Geometry: final body of the model. Coordinates: model frame, mm. Round coordinates to 2 decimals unless told otherwise and drop trailing zeros. Order: outer loops, then holes, each group sorted by start corner. A loop starts at its lowest first (then second) coordinate and runs counter-clockwise, first axis right, second up. Notation, with made-up numbers: (89, 1.25) - (143, 1.25) arc R23 ccw to (143, 32.25) - close; hole circle Ø9 at (-20.75, 11). An arc over 180 degrees is marked (long way). Put each result on its own line as item: value. Start each with the question number.
(1) Pin query (flat end, axial travel): P1, Ø12, axis at y = 0, z = 9, coming from the -X side; P2, Ø10, axis at y = 8.5, z = 65.5, coming from the -X side. Return the tip coordinate at first contact, or that it passes through.
(2) Section C-C (z = 9). Output: boundary loops of the cut face in (x, y).
(3) Material intervals for L1, parallel to Y at x = 3.5, z = -61; L2, parallel to Z at x = 5.5, y = -32.5; L3, parallel to Y at x = 6.5, z = 9, sorted ascending. Write a range as [from, to].
(4) Pull-direction query (Y, two-part tool) for faces 1 (the face through (4.93, -38.58, -53.06)), 2 (the face through (5, 0, 19)), 3 (the face through (0, 14, 1)), 4 (the face through (5, 60, 1)); classes: released by +Y, released by -Y, zero draft, split by the parting line, or undercut.
(5) Section D-D (x = 5.5). Output: boundary loops of the cut face in (y, z), and give its area (3 significant figures).
(6) Section A-A (z = -61). Output: boundary loops of the cut face in (x, y).
(7) Section B-B (y = 32.5). Output: boundary loops of the cut face in (x, z), and give its area (3 significant figures).
from build123d import *

# Parameters (mm, degrees)
SKETCH1_W               = 172
SKETCH1_H               = 120
BOSS_EXTRUDE1_DEPTH     = 10
CUT_EXTRUDE1_DEPTH      = 106.337552658
CUT_EXTRUDE1_DEPTH_BACK = 106.337552658
SKETCH2_R               = 10


with BuildPart() as part:
    # Sketch1 → Boss-Extrude1 (new body)
    with BuildSketch(Plane(origin=(0, 0, 0), x_dir=(0, 0, -1), z_dir=(1, 0, 0))):
        Rectangle(SKETCH1_W, SKETCH1_H)
    extrude(amount=BOSS_EXTRUDE1_DEPTH)

    # Sketch2 → Cut-Extrude1 (cut, two sides: drawn at the far end of the back side and taken through both)
    with BuildSketch(Plane(origin=(10, 0, 0), x_dir=(0, 0, -1), z_dir=(1, 0, 0)).offset(-CUT_EXTRUDE1_DEPTH_BACK)):
        with Locations((-9, 0)):
            Circle(SKETCH2_R)
        with Locations((61, 32.5)):
            Circle(SKETCH2_R)
        with Locations((61, -32.5)):
            Circle(SKETCH2_R)
    extrude(amount=CUT_EXTRUDE1_DEPTH + CUT_EXTRUDE1_DEPTH_BACK, mode=Mode.SUBTRACT)


solid = part.part
Checks:
1. P1: passes through
1. P2: stops at x = 0
2. outline: (0, -60) - (10, -60) - (10, -10) - (0, -10) - close; (0, 10) - (10, 10) - (10, 60) - (0, 60) - close
3. L1: y = [-60, -42.5], [-22.5, 22.5], [42.5, 60]
3. L2: z = [-86, -71], [-51, 86]
3. L3: y = [-60, -10], [10, 60]
4. face 1: undercut
4. face 2: undercut
4. face 3: zero draft
4. face 4: released by +Y
5. outline: (-60, -86) - (60, -86) - (60, 86) - (-60, 86) - close; hole circle Ø20 at (-32.5, -61); hole circle Ø20 at (0, 9); hole circle Ø20 at (32.5, -61)
5. area: 19,700 mm²
6. outline: (0, -60) - (10, -60) - (10, -42.5) - (0, -42.5) - close; (0, -22.5) - (10, -22.5) - (10, 22.5) - (0, 22.5) - close; (0, 42.5) - (10, 42.5) - (10, 60) - (0, 60) - close
7. outline: (0, -86) - (10, -86) - (10, -71) - (0, -71) - close; (0, -51) - (10, -51) - (10, 86) - (0, 86) - close
7. area: 1,520 mm²
